Read the model definition and answer for the solid it produces. Units are mm, in the model's axes. A direction names the side the tool comes from. Coordinates: 2 decimals unless noted, no trailing zeros. Write each loop counter-clockwise with the first axis right and the second up, starting at its lowest first coordinate (ties: lowest second). Pieces come first, ordered by that corner, then holes.
Item 1: Section C-C (x = 22) is taken. Give the vertices of the cut face in (y, z).
Item 2: Section A-A (z = 15) is taken. Give the vertices of the cut face in (x, y), then the cut area to 3 significant figures.
Item 3: Straight lines are drawn through the part: probe 1 along X at (y, z) = (-11.75, 17); probe 2 along Z at (x, y) = (-18, -2.25); probe 3 along Y at (x, z) = (-13, 1.5). For each, find the intervals that lie inside material, in ascending order.
Item 4: Section D-D (y = -1.75) is taken. Give the vertices of the cut face in (x, z).
Item 5: Each of these flat-tipped pins is pushed along its axis until it touches: P1, Ø1.5, axis at x = 10.5, y = -14.5, coming from the +Z side; P2, Ø12.5, axis at x = 34.5, y = -16.5, coming from the -Z side. Where does it stop, or does it pass through?
Item 6: Section B-B (y = -12.75) is taken. Give the vertices of the cut face in (x, z).
Item 7: A tool of negligible diameter and unlimited length cuts with its end or side. For faces 1 (the face through (38, -13, -12.7)), 2 (the face through (0.711, -19.092, 1.304)), 3 (the face through (0, -13, 12.7)), from which of +Z, -Z, +X, -X, +Y, -Y can it reach the whole face along a straight path? Write none if from no direction.
Item 8: Determine the mould class of faces 4 (the face through (-50.8, -13, -6)), 5 (the face through (25.4, -13, 19)), 6 (the face through (25.4, -13, -19)), 7 (the face through (-1, -25.4, 0)) for opening direction X: released by +X, released by -X, zero draft, split by the parting line, or undercut.
from build123d import *

# Parameters (mm, degrees)
F0_W     = 101.6
F0_H     = 50.8
F1_DEPTH = 25.4
F2_W     = 25.4
F2_H     = 12.7
F3_DEPTH = 25.401
F4_R     = 6.35
F5_DEPTH = 101.601
F6_W     = 50.8
F6_H     = 12.7
F7_DEPTH = 25.401


with BuildPart() as f1:
    # F0 (on Front) → F1 (new body)
    with BuildSketch(Plane.XZ):
        Rectangle(F0_W, F0_H)
    extrude(amount=F1_DEPTH)

    # F2 (on face) → F3 (cut, through all)
    with BuildSketch(Plane.XZ.offset(25.4)):
        with Locations((38.1, -19.05)):
            Rectangle(F2_W, F2_H)
    extrude(amount=-F3_DEPTH, mode=Mode.SUBTRACT)

    # F4 (on face) → F5 (cut, through all)
    with BuildSketch(Plane.YZ.offset(50.8)):
        with Locations((-12.748572, 1.024565)):
            Circle(F4_R)
    extrude(amount=-F5_DEPTH, mode=Mode.SUBTRACT)

    # F6 (on face) → F7 (cut, through all)
    with BuildSketch(Plane.XZ.offset(25.4)):
        with Locations((0, 19.05)):
            Rectangle(F6_W, F6_H)
    extrude(amount=-F7_DEPTH, mode=Mode.SUBTRACT)


solid = f1.part
Established:
1. outline: (-25.4, -25.4) - (0, -25.4) - (0, 12.7) - (-25.4, 12.7) - close; hole circle Ø12.7 at (-12.75, 1.02)
2. outline: (-50.8, -25.4) - (-25.4, -25.4) - (-25.4, 0) - (-50.8, 0) - close; (25.4, -25.4) - (50.8, -25.4) - (50.8, 0) - (25.4, 0) - close
2. area: 1,290 mm2
3. probe 1: x = -50.8 to -25.4, 25.4 to 50.8
3. probe 2: z = -25.4 to 12.7
3. probe 3: y = -25.4 to -19.08, -6.42 to 0
4. outline: (-50.8, -25.4) - (25.4, -25.4) - (25.4, -12.7) - (50.8, -12.7) - (50.8, 25.4) - (25.4, 25.4) - (25.4, 12.7) - (-25.4, 12.7) - (-25.4, 25.4) - (-50.8, 25.4) - close
5. P1: stops at z = 12.7
5. P2: stops at z = -12.7
6. outline: (-50.8, -25.4) - (25.4, -25.4) - (25.4, -12.7) - (50.8, -12.7) - (50.8, -5.33) - (-50.8, -5.33) - close; (-50.8, 7.37) - (50.8, 7.37) - (50.8, 25.4) - (25.4, 25.4) - (25.4, 12.7) - (-25.4, 12.7) - (-25.4, 25.4) - (-50.8, 25.4) - close
7. face 1: -Z, +X, +Y, -Y
7. face 2: +X, -X
7. face 3: +Z, +Y, -Y
8. face 4: released by -X
8. face 5: undercut
8. face 6: released by +X
8. face 7: zero draft
